Input: part model. Units: mm. Frame: model coordinates. A direction names the side the tool comes from. Coordinates: 2 decimals unless noted, no trailing zeros. Write each loop counter-clockwise with the first axis right and the second up, starting at its lowest first coordinate (ties: lowest second). Pieces come first, ordered by that corner, then holes. Notation, with made-up numbers: (71, 30) - (78, 30) arc R8 ccw to (78, 40) - close; hole circle Ø11 at (75, -11.5). An arc over 180 degrees is marked (long way). Put each result on its own line as item: value. Start each with the question number.
1. Line query: line 1 (Y direction, x = -13, z = -3.5); line 2 (X direction, y = -82, z = -4.5); line 3 (Z direction, x = -30, y = 111.5). Output: solid intervals per line, ascending.
2. Cut plane A-A, the plane x = -211. Return loops of the section in (y, z).
3. Cut plane D-D, the plane y = -117. Return loops of the section in (x, z).
4. Pull-direction query (Y, two-part tool) for faces 4 (the flat face through (-123, 2, 13.439)), 5 (the cylindrical face through (-123.285, -125.011, 8.782)), 6 (the flat face through (-123.25, 133.25, -5.74)), 7 (the flat face through (0, -2, -1)); classes: released by +Y, released by -Y, zero draft, split by the parting line, or undercut.
5. Access query for faces 1 (the flat face through (-123.28, -131.04, -10.96)), 2 (the cylindrical face through (-123.25, -126.709, 10.617)), 3 (the flat face through (-123.29, 130.83, -7.2)). Directions: +Z, -Z, +X, -X, +Y, -Y. A direction counts if a zero-diameter tool reaches every point of the face in a straight line with its end or side. Return the directions, or none.
6. Cut plane C-C, the plane z = 2. Return loops of the section in (x, y).
7. Cut plane B-B, the plane y = 13.5. Return loops of the section in (x, z), and give its area (4 significant figures).
8. Pin query (flat end, axial travel): pin 1 (12 mm diameter, centred on x = -61, z = 3, fed in from -Y); pin 2 (12 mm diameter, centred on x = -100.5, y = -60.5, fed in from -Z); pin 3 (10 mm diameter, centred on x = -114.5, z = 0.5, fed in from -Y). Return the tip coordinate at first contact, or that it passes through.
from build123d import *

# Parameters (mm, degrees)
F1_DEPTH = 250
F2_T     = -2.5
F3_W     = 245
F3_H     = 8
F4_DEPTH = 267.5780191142
F6_DEPTH = 245


with BuildPart() as f1:
    # F0 (on Right) → F1 (new body)
    with BuildSketch(Plane.YZ):
        with BuildLine():
            Line((-134.0000000003, -19.0613823906), (133.9999999997, -19.0613823906))
            Line((133.9999999997, -19.0613823906), (133.0930686257, -2.9381579633))
            ThreePointArc((133.0930686257, -2.9381579633), (126.8639122094, 10.4724486347), (113.1246343635, 15.9386176094))
            Line((113.1246343635, 15.9386176094), (-113.1246343631, 15.9386176094))
            ThreePointArc((-113.1246343631, 15.9386176094), (-126.8639122086, 10.4724486351), (-133.0930686253, -2.9381579622))
            Line((-133.0930686253, -2.9381579622), (-134.0000000003, -19.0613823906))
        make_face()
    extrude(amount=-F1_DEPTH)

    # F2
    f2_openings = [f1.faces().sort_by_distance(p)[0] for p in [
        (-125, 0, -19.061382),
    ]]
    offset(amount=F2_T, openings=f2_openings)

    # F3 (on face) → F4 (cut, through all)
    with BuildSketch(Plane(origin=(0, 132.5085319634, 7.4536049229), x_dir=(-1, 0, 0), z_dir=(0, 0.9984217131, 0.0561612214))):
        with Locations((125, -22.5569017233)):
            Rectangle(F3_W, F3_H)
    extrude(amount=-F4_DEPTH, mode=Mode.SUBTRACT)

    # F5 (on face) → F6 (join)
    with BuildSketch(Plane.YZ.offset(-247.5)):
        with BuildLine():
            Line((133.6349520609, -12.5716412553), (133.5647505342, -11.3236141139))
            ThreePointArc((133.5647505342, -11.3236141139), (130.0312736901, -15.2783001182), (133.9859596944, -18.8117769623))
            Line((133.9859596944, -18.8117769623), (133.9157581677, -17.5637498209))
            ThreePointArc((133.9157581677, -17.5637498209), (131.2793008315, -15.2080985915), (133.6349520609, -12.5716412553))
        make_face()
        with BuildLine():
            ThreePointArc((133.9859596944, -18.8117769623), (136.5004484315, -17.6438101342), (137.5253551143, -15.0676955381))
            ThreePointArc((137.5253551143, -15.0676955381), (136.3514697104, -12.3426022209), (133.5647505342, -11.3236141139))
            Line((133.5647505342, -11.3236141139), (133.6349520609, -12.5716412553))
            ThreePointArc((133.6349520609, -12.5716412553), (135.492764845, -13.25096666), (136.2753551143, -15.0676955381))
            ThreePointArc((136.2753551143, -15.0676955381), (135.5920839925, -16.7851052689), (133.9157581677, -17.5637498209))
            Line((133.9157581677, -17.5637498209), (133.9859596944, -18.8117769623))
        make_face()
    extrude(amount=F6_DEPTH)


solid = f1.part
Report:
1. line 1: y = -133.12 to -130.62, 130.62 to 133.12
1. line 2: x = -250 to -247.5, -2.5 to 0
1. line 3: z = 13.44 to 15.94
2. outline: (-134, -19.06) - (-131.5, -19.06) - (-130.6, -3.08) arc R17.5 cw to (-113.12, 13.44) - (113.12, 13.44) arc R17.5 cw to (130.6, -3.08) - (131.05, -11.21) - (133.55, -11.07) - (133.09, -2.94) arc R20 ccw to (113.12, 15.94) - (-113.12, 15.94) arc R20 ccw to (-133.09, -2.94) - close; circle Ø7.5 at (133.78, -15.07); hole circle Ø5 at (133.78, -15.07)
3. outline: (-250, -19.06) - (-247.5, -19.06) - (-247.5, 13) - (-2.5, 13) - (-2.5, -19.06) - (0, -19.06) - (0, 15.56) - (-250, 15.56) - close
4. face 4: undercut
4. face 5: undercut
4. face 6: released by +Y
4. face 7: zero draft
5. face 1: -Z
5. face 2: +Z, +X, -X, -Y
5. face 3: none
6. outline: (-250, -132.18) - (0, -132.18) - (0, 132.18) - (-250, 132.18) - close; hole (-247.5, -129.54) - (-2.5, -129.54) - (-2.5, 129.54) - (-247.5, 129.54) - close
7. outline: (-250, -19.06) - (-247.5, -19.06) - (-247.5, 13.44) - (-2.5, 13.44) - (-2.5, -19.06) - (0, -19.06) - (0, 15.94) - (-250, 15.94) - close
7. area: 787.5 mm^2
8. pin 1: stops at y = -133.1
8. pin 2: stops at z = 13.44
8. pin 3: stops at y = -133.18
